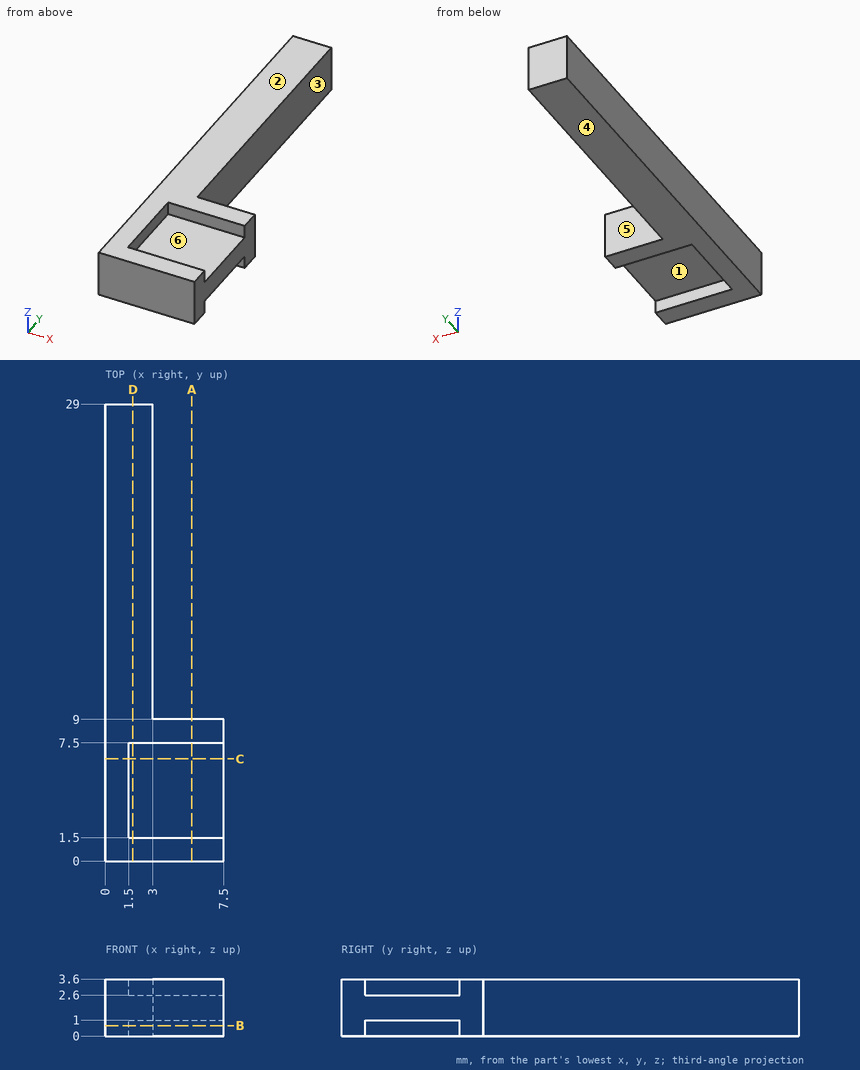
The figure shows three views and two pictorial views of one solid part (mm, origin at its lowest corner). Answer the questions. A direction names the side the tool comes from. Coordinates: 2 decimals unless noted, no trailing zeros. Write each loop counter-clockwise with the first axis right and the second up, starting at its lowest first coordinate (ties: lowest second). Pieces come first, ordered by that corner, then holes. Notation, with made-up numbers: (-36.5, 30.5) -> (-0.5, 30.5) arc R38 cw to (-0.5, 69.5) -> close; hole circle Ø1 at (53, -15.75). An arc over 180 degrees is marked (long way). Return JSON: item names as keys, results as strings.
1. A cutting plane is placed at A-A (x = 5.5). Determine the outline of the cut face in (y, z), and give its area (3 significant figures).
Found:
{"outline": "(0, 0) -> (1.5, 0) -> (1.5, 1) -> (7.5, 1) -> (7.5, 0) -> (9, 0) -> (9, 3.6) -> (7.5, 3.6) -> (7.5, 2.6) -> (1.5, 2.6) -> (1.5, 3.6) -> (0, 3.6) -> close", "area": "20.4 mm2"}
2. A cutting plane is placed at C-C (y = 6.5). Determine the outline of the cut face in (x, z).
Found:
{"outline": "(0, 0) -> (1.5, 0) -> (1.5, 1) -> (7.5, 1) -> (7.5, 2.6) -> (1.5, 2.6) -> (1.5, 3.6) -> (0, 3.6) -> close"}
3. Find the intervals of material crossed by line 1 along Y through (x, z) = (5.25, 2.7); line 2 along Y through (x, z) = (1.75, 0.55); line 3 along Y through (x, z) = (5.5, 1.5), in increasing order. Write a range as from..to.
Found:
{"line 1": "0..1.5, 7.5..9", "line 2": "0..1.5, 7.5..29", "line 3": "0..9"}
4. Each of these flat-tipped pins is pushed along its axis until it touches: P1, Ø1.1, axis at y = 21.5, z = 1, coming from the +X side; P2, Ø2, axis at x = 3.5, y = 5, coming from the +Z side. Where does it stop, or does it pass through?
Found:
{"P1": "x = 3", "P2": "z = 2.6"}
5. A cutting plane is placed at B-B (z = 0.65). Determine the outline of the cut face in (x, y).
Found:
{"outline": "(0, 0) -> (7.5, 0) -> (7.5, 1.5) -> (1.5, 1.5) -> (1.5, 7.5) -> (7.5, 7.5) -> (7.5, 9) -> (3, 9) -> (3, 29) -> (0, 29) -> close"}
6. Determine the mould class of the marked faces 4, 5 and 6 for opening direction Y: pulls with the +Y half, pulls with the -Y half, needs draft (parallel to the pull), parting line crosses it, or undercut.
Found:
{"face 4": "needs draft", "face 5": "pulls with the +Y half", "face 6": "undercut"}
7. A tool of negligible diameter and unlimited length cuts with its end or side. For the marked faces 1, 2 and 3, from which of +Z, -Z, +X, -X, +Y, -Y can it reach the whole face along a straight path? Write none if from no direction.
Found:
{"face 1": "-Z, +X", "face 2": "+Z, +X, -X, +Y, -Y", "face 3": "+Z, -Z, +X, +Y"}
8. A cutting plane is placed at D-D (x = 1.75). Determine the outline of the cut face in (y, z), and give its area (3 significant figures).
Found:
{"outline": "(0, 0) -> (1.5, 0) -> (1.5, 1) -> (7.5, 1) -> (7.5, 0) -> (29, 0) -> (29, 3.6) -> (7.5, 3.6) -> (7.5, 2.6) -> (1.5, 2.6) -> (1.5, 3.6) -> (0, 3.6) -> close", "area": "92.4 mm2"}
